Model file for the job. Use its own axes, mm. A direction names the side the tool comes from. Give positions to 0.01 mm unless a question says otherwise; leave off trailing zeros. Write each loop counter-clockwise with the first axis right and the second up, starting at its lowest first coordinate (ties: lowest second). Pieces come first, ordered by that corner, then holes. Notation, with made-up numbers: (-35, 74.25) - (21, 74.25) arc R21 ccw to (21, 78.25) - close; hole circle Ø3 at (-14.75, 11.25). An arc over 180 degrees is marked (long way). Use CSV: the item, a comma, the result in double quotes.
from build123d import *

# Parameters (mm, degrees)
SKETCH1_R                                     = 37.5
BOSS_EXTRUDE1_DEPTH                           = 3
SKETCH1_3_R                                   = 35
BOSS_EXTRUDE2_DEPTH                           = 12
SKETCH13_R                                    = 16
CUT_EXTRUDE6_DEPTH                            = 55.373706881
BOSS_EXTRUDE9_DEPTH                           = 2
SKETCH25_R                                    = 7.5
BOSS_EXTRUDE10_DEPTH                          = 15
SKETCH26_R                                    = 5
CUT_EXTRUDE9_DEPTH                            = 5
CBORE_FOR_M3_PAN_HEAD_MACHINE_SCREW1_AT_COUNT = 2
CBORE_FOR_M3_PAN_HEAD_MACHINE_SCREW1_AT_PITCH = 46.765371804
CBORE_FOR_M3_PAN_HEAD_MACHINE_SCREW1_2_COUNT  = 2
CBORE_FOR_M3_PAN_HEAD_MACHINE_SCREW1_2_PITCH  = 46.765371804
SKETCH29_R                                    = 1.75
CUT_EXTRUDE10_DEPTH                           = 56.691112397
SKETCH31_R                                    = 16.05
BOSS_EXTRUDE11_DEPTH                          = 50
SKETCH32_R                                    = 18
SKETCH32_R_2                                  = 16
BOSS_EXTRUDE12_DEPTH                          = 1.11


with BuildPart() as part:
    # Sketch1 → Boss-Extrude1 (new body)
    with BuildSketch(Plane(origin=(0, 0, 0), x_dir=(1, 0, 0), z_dir=(0, 1, 0))):
        with Locations(Location((0, 0, 0), (0, 0, 270))):
            Circle(SKETCH1_R)
    extrude(amount=BOSS_EXTRUDE1_DEPTH)

    # Sketch1_3 → Boss-Extrude2 (add)
    with BuildSketch(Plane(origin=(0, 0, 0), x_dir=(1, 0, 0), z_dir=(0, 1, 0))):
        with Locations(Location((0, 0, 0), (0, 0, 270))):
            Circle(SKETCH1_3_R)
    extrude(amount=BOSS_EXTRUDE2_DEPTH)

    # Sketch13 → Cut-Extrude6 (cut, through all)
    with BuildSketch(Plane(origin=(0, 12, 0), x_dir=(1, 0, 0), z_dir=(0, 1, 0))):
        with Locations(Location((0, 0, 0), (0, 0, 270))):
            Circle(SKETCH13_R)
    extrude(amount=-CUT_EXTRUDE6_DEPTH, mode=Mode.SUBTRACT)

    # Sketch24 → Boss-Extrude9 (add)
    with BuildSketch(Plane(origin=(0, 12, 0), x_dir=(1, 0, 0), z_dir=(0, 1, 0))):
        with BuildLine():
            ThreePointArc((5.813043417, 34.513888889), (0, 35), (-5.813043417, 34.513888889))
            ThreePointArc((-5.813043417, 34.513888889), (0, 17.5), (5.813043417, 34.513888889))
        make_face()
        with BuildLine():
            ThreePointArc((-26.983382853, -22.291187717), (-15.155444566, -8.75), (-32.79642627, -12.222701172))
            ThreePointArc((-32.79642627, -12.222701172), (-30.310889132, -17.5), (-26.983382853, -22.291187717))
        make_face()
        with BuildLine():
            ThreePointArc((26.983382853, -22.291187717), (30.310889132, -17.5), (32.79642627, -12.222701172))
            ThreePointArc((32.79642627, -12.222701172), (15.155444566, -8.75), (26.983382853, -22.291187717))
        make_face()
    extrude(amount=BOSS_EXTRUDE9_DEPTH)

    # Sketch25 → Boss-Extrude10 (add)
    with BuildSketch(Plane(origin=(0, 14, 0), x_dir=(1, 0, 0), z_dir=(0, 1, 0))):
        with Locations(Location((0, 27, 0), (0, 0, 270))):
            Circle(SKETCH25_R)
        with Locations(Location((23.382685902, -13.5, 0), (0, 0, 270))):
            Circle(SKETCH25_R)
        with Locations(Location((-23.382685902, -13.5, 0), (0, 0, 270))):
            Circle(SKETCH25_R)
    extrude(amount=BOSS_EXTRUDE10_DEPTH)

    # Sketch26 → Cut-Extrude9 (cut)
    with BuildSketch(Plane(origin=(0, 29, 0), x_dir=(1, 0, 0), z_dir=(0, 1, 0))):
        with Locations(Location((0, 27, 0), (0, 0, 270))):
            Circle(SKETCH26_R)
        with Locations(Location((23.382685902, -13.5, 0), (0, 0, 270))):
            Circle(SKETCH26_R)
        with Locations(Location((-23.382685902, -13.5, 0), (0, 0, 270))):
            Circle(SKETCH26_R)
    extrude(amount=-CUT_EXTRUDE9_DEPTH, mode=Mode.SUBTRACT)

    # Sketch28 → CBORE for M3 Pan Head Machine Screw1 (revolve, cut)
    with BuildSketch(Plane(origin=(0, 0, -27), x_dir=(0, 0, -1), z_dir=(1, 0, 0))):
        Polygon((0, 0), (0, 29), (1.8, 29), (1.8, 2.4), (3.5, 2.4), (3.5, 0.025), (3.525, 0), align=None)
    cbore_for_m3_pan_head_machine_screw1 = revolve(axis=Axis((0, -6.35, -27), (0, 1, 0)), mode=Mode.SUBTRACT)

    # CBORE for M3 Pan Head Machine Screw1 at: CBORE for M3 Pan Head Machine Screw1 ×2
    with Locations(*[Vector(-0.5000000000000369, 0, 0.8660254037844174) * (i * CBORE_FOR_M3_PAN_HEAD_MACHINE_SCREW1_AT_PITCH) for i in range(1, CBORE_FOR_M3_PAN_HEAD_MACHINE_SCREW1_AT_COUNT)]):
        add(cbore_for_m3_pan_head_machine_screw1, mode=Mode.SUBTRACT)

    # CBORE for M3 Pan Head Machine Screw1 2: CBORE for M3 Pan Head Machine Screw1 ×2
    with Locations(*[Vector(0.49999999999996353, 0, 0.8660254037844598) * (i * CBORE_FOR_M3_PAN_HEAD_MACHINE_SCREW1_2_PITCH) for i in range(1, CBORE_FOR_M3_PAN_HEAD_MACHINE_SCREW1_2_COUNT)]):
        add(cbore_for_m3_pan_head_machine_screw1, mode=Mode.SUBTRACT)

    # Sketch29 → Cut-Extrude10 (cut, through all)
    with BuildSketch(Plane(origin=(0, 12, 0), x_dir=(1, 0, 0), z_dir=(0, 1, 0))):
        with Locations(Location((23.382685902, 13.5, 0), (0, 0, 270))):
            Circle(SKETCH29_R)
        with Locations(Location((0, -27, 0), (0, 0, 270))):
            Circle(SKETCH29_R)
        with Locations(Location((-23.382685902, 13.5, 0), (0, 0, 270))):
            Circle(SKETCH29_R)
    extrude(amount=-CUT_EXTRUDE10_DEPTH, mode=Mode.SUBTRACT)



with BuildPart() as body_2:
    # Sketch31 → Boss-Extrude11 (new body)
    with BuildSketch(Plane.XZ):
        with Locations(Location((0, 0, 0), (0, 0, 270))):
            Circle(SKETCH31_R)
    extrude(amount=BOSS_EXTRUDE11_DEPTH)


with BuildPart() as part_1:
    add(part.part)

    add(body_2.part)  # Boss-Extrude12 merges body 2
    # Sketch32 → Boss-Extrude12 (add)
    with BuildSketch(Plane.XZ):
        with Locations(Location((0, 0, 0), (0, 0, 90))):
            Circle(SKETCH32_R)
        with Locations(Location((0, 0, 0), (0, 0, 90))):
            Circle(SKETCH32_R_2, mode=Mode.SUBTRACT)
    extrude(amount=BOSS_EXTRUDE12_DEPTH)


solid = part_1.part
(1) Saw through at B-B, the plane z = 27. List the corners of the cut face in (x, y).
Checked values:
outline,"(-26.02, 0) - (-1.75, 0) - (-1.75, 12) - (-22.27, 12) - (-22.27, 3) - (-26.02, 3) - close; (1.75, 0) - (26.02, 0) - (26.02, 3) - (22.27, 3) - (22.27, 12) - (1.75, 12) - close"
(2) Flat gauge pins, fed straight in: P1, Ø2, axis at x = 21.5, z = 12.5, coming from the -Y side; P2, Ø4, axis at x = -23.38, z = -13.5, coming from the -Y side; P3, Ø2, axis at y = 15.5, z = 3.5, coming from the +X side; P4, Ø10, axis at x = 29.5, y = 0, coming from the -Z side. Where does each tip first touch, or does it go through?
Checked values:
P1,"stops at y = 2.4"
P2,"stops at y = 0"
P3,"passes through"
P4,"stops at z = -28.39"
(3) Saw through at C-C, the plane z = -13.5. List the corners of the cut face in (x, y).
Checked values:
outline,"(-34.99, 0) - (-25.13, 0) - (-25.13, 12) - (-32.29, 12) - (-32.29, 3) - (-34.99, 3) - close; (-21.63, 0) - (-11.91, 0) - (-11.91, -1.11) - (-8.68, -1.11) - (-8.68, -50) - (8.68, -50) - (8.68, -1.11) - (11.91, -1.11) - (11.91, 0) - (21.63, 0) - (21.63, 12) - (8.59, 12) - (8.59, 0) - (-8.59, 0) - (-8.59, 12) - (-21.63, 12) - close; (25.13, 0) - (34.99, 0) - (34.99, 3) - (32.29, 3) - (32.29, 12) - (25.13, 12) - close"
(4) Saw through at D-D, the plane x = 0. Count the separate pieces of the cut face and the enclosed holes in it, then the cut area to 3 significant figures.
Checked values:
separate pieces,"3"
enclosed holes,"0"
area,"2,150 mm^2"
(5) Saw through at A-A, the plane z = 0. List the corners of the cut face in (x, y).
Checked values:
outline,"(-37.5, 0) - (-18, 0) - (-18, -1.11) - (-16.05, -1.11) - (-16.05, -50) - (16.05, -50) - (16.05, -1.11) - (18, -1.11) - (18, 0) - (37.5, 0) - (37.5, 3) - (35, 3) - (35, 12) - (16, 12) - (16, 0) - (-16, 0) - (-16, 12) - (-35, 12) - (-35, 3) - (-37.5, 3) - close"
(6) 3-axis set-ups, long thin cutter, end or side, ignore diameter. For faces 1 (the face through (0.08, 6.08, 25.25)), 2 (the face through (-26, 24, 13)), 3 (the face through (26.488, 1.196, 11.885)): which of +Z, -Z, +X, -X, +Y, -Y reach the whole face in a straight line?
Checked values:
face 1,"+Y, -Y"
face 2,"+Y"
face 3,"-Y"
(7) Wall check: probe 1 along X at (y, z) = (27, 13); probe 2 along X at (y, z) = (9.75, 0); probe 3 along Y at (x, z) = (5, -24). Give the ranges that are in metal, low to high. Write a range as [from, to].
Checked values:
probe 1,"x = [-30.87, -28.36], [-18.41, -15.9], [15.9, 18.41], [28.36, 30.87]"
probe 2,"x = [-35, -16], [16, 35]"
probe 3,"y = [0, 29]"
(8) Pull direction Z, two halves, no side cores. Call faces 4 (the face through (-16, 14, 11)), 5 (the face through (-2, 24, -27)), 6 (the face through (-5.407, -0.547, 17.169)): released by +Z, released by -Z, zero draft, split by the parting line, or undercut.
Checked values:
face 4,"zero draft"
face 5,"undercut"
face 6,"split by the parting line"
